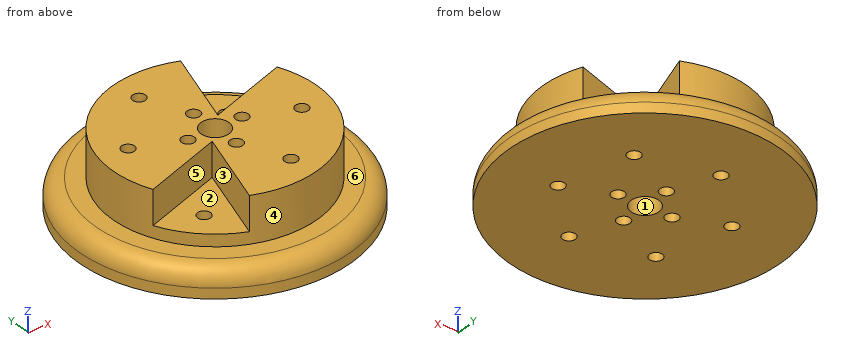
from build123d import *

# Parameters (mm, degrees)
F0_R     = 30
F0_R_2   = 1.9
F0_R_3   = 4.075
F1_DEPTH = 21.5
F0_R_4   = 40
F2_DEPTH = 8
F3_R     = 1.9
F4_DEPTH = 10
F5_R     = 5


with BuildPart() as f1:
    # F0 (on Top) → F1 (new body)
    with BuildSketch(Plane.XY):
        Circle(F0_R)
        with Locations((-15.5563491861, -15.5563491861)):
            Circle(F0_R_2, mode=Mode.SUBTRACT)
        with Locations((5.6940189923, -21.2503681784)):
            Circle(F0_R_2, mode=Mode.SUBTRACT)
        with Locations((0, -8)):
            Circle(F0_R_2, mode=Mode.SUBTRACT)
        with Locations((21.2503681784, -5.6940189923)):
            Circle(F0_R_2, mode=Mode.SUBTRACT)
        with Locations((-21.2503681784, 5.6940189923)):
            Circle(F0_R_2, mode=Mode.SUBTRACT)
        with Locations((-8, 0)):
            Circle(F0_R_2, mode=Mode.SUBTRACT)
        with Locations((-5.6940189923, 21.2503681784)):
            Circle(F0_R_2, mode=Mode.SUBTRACT)
        Circle(F0_R_3, mode=Mode.SUBTRACT)
        with Locations((8, 0)):
            Circle(F0_R_2, mode=Mode.SUBTRACT)
        with Locations((0, 8)):
            Circle(F0_R_2, mode=Mode.SUBTRACT)
        with Locations((15.5563491861, 15.5563491861)):
            Circle(F0_R_2, mode=Mode.SUBTRACT)
    extrude(amount=F1_DEPTH)

    # F0 (on Top) → F2 (join)
    with BuildSketch(Plane.XY):
        Circle(F0_R_4)
        Circle(F0_R, mode=Mode.SUBTRACT)
    extrude(amount=F2_DEPTH)

    # F3 (on face) → F4 (cut)
    with BuildSketch(Plane.XY.offset(21.5)):
        with BuildLine():
            Line((-11.6844405683, -27.6310305382), (-4, -4))
            Line((-4, -4), (-27.6310305382, -11.6844405683))
            ThreePointArc((-27.6310305382, -11.6844405683), (-21.2132034356, -21.2132034356), (-11.6844405683, -27.6310305382))
        make_face()
        with Locations((-15.5563491861, -15.5563491861)):
            Circle(F3_R, mode=Mode.SUBTRACT)
        with BuildLine():
            ThreePointArc((27.6310305382, 11.6844405683), (21.2132034356, 21.2132034356), (11.6844405683, 27.6310305382))
            Line((11.6844405683, 27.6310305382), (4, 4))
            Line((4, 4), (27.6310305382, 11.6844405683))
        make_face()
        with Locations((15.5563491861, 15.5563491861)):
            Circle(F3_R, mode=Mode.SUBTRACT)
    extrude(amount=-F4_DEPTH, mode=Mode.SUBTRACT)

    # F5
    f5_edges = [f1.edges().sort_by_distance(p)[0] for p in [
        (-40, 0, 8),
    ]]
    fillet(f5_edges, radius=F5_R)


solid = f1.part
Input: part model. Units: mm. Frame: model coordinates. Face numbers are marked on the shaded views. A direction names the side the tool comes from. Round coordinates to 2 decimals unless told otherwise and drop trailing zeros. Loops run counter-clockwise (first coordinate to the right, second up) from the corner with the lowest first, then second, coordinate; pieces in that order, holes last. Notation, with made-up numbers: (-16.5, 48.25) -> (39.5, 48.25) arc R12 cw to (39.5, 59.25) -> close; hole circle Ø6 at (26.25, -19.5). An arc over 180 degrees is marked (long way). Answer as a JSON object with one key per item and string values. Group by question number.
1) Pin query (flat end, axial travel): pin 1 (1.5 mm diameter, centred on x = -12.5, z = 16.5, fed in from +Y); pin 2 (4 mm diameter, centred on x = -28.5, z = 3.5, fed in from +Y); pin 3 (10 mm diameter, centred on x = -15, z = 3, fed in from +Y). Return the tip coordinate at first contact, or that it passes through.
2) Ray query, L1, parallel to Z at x = 30, y = -13.5; L2, parallel to Y at x = -2, z = 4.5; L3, parallel to Y at x = 0, z = 5 (3 decimals). Return the intervals inside material, ascending.
3) Reachability of the marked faces 1 and 2 from +Z, -Z, +X, -X, +Y, -Y: full face, straight path, thin tool, end or side. Return the list, or none.
4) Draft query along X for the marked faces 3, 4, 5 and 6. Return one class per face: +X half, -X half, draft (parallel to the pull), parting line (faces both ways), or undercut.
5) Section query C-C on z = 9.5. State how many separate pieces and enclosed holes the cut face has, plus the area to 3 significant figures.
6) Section query A-A on y = 0. Output: boundary loops of the cut face in (x, z) (3 decimals).
Reply:
{
 "1": {"pin 1": "stops at y = 27.6", "pin 2": "stops at y = 29.94", "pin 3": "stops at y = 38.73"},
 "2": {"L1": "z = 0 to 8", "L2": "y = -39.72 to -3.55, 3.55 to 39.72", "L3": "y = -39.583 to -9.9, -6.1 to -4.075, 4.075 to 6.1, 9.9 to 39.583"},
 "3": {"face 1": "+Z, -Z", "face 2": "+Z"},
 "4": {"face 3": "undercut", "face 4": "parting line", "face 5": "undercut", "face 6": "draft"},
 "5": {"separate pieces": "1", "enclosed holes": "11", "area": "2,660 mm2"},
 "6": {"outline": "(-40, 0) -> (-9.9, 0) -> (-9.9, 21.5) -> (-30, 21.5) -> (-30, 8) -> (-35, 8) arc R5 ccw to (-40, 3) -> close; (-6.1, 0) -> (-4.075, 0) -> (-4.075, 21.5) -> (-6.1, 21.5) -> close; (4.075, 0) -> (6.1, 0) -> (6.1, 21.5) -> (4.075, 21.5) -> close; (9.9, 0) -> (40, 0) -> (40, 3) arc R5 ccw to (35, 8) -> (30, 8) -> (30, 21.5) -> (9.9, 21.5) -> close"}
}
